Can you work these out from the model? Positions are in its coordinate system, mm. Face numbers are marked on the shaded views. A direction names the side the tool comes from. Round coordinates to 2 decimals unless told otherwise and drop trailing zeros. Loops run counter-clockwise (first coordinate to the right, second up) from the corner with the lowest first, then second, coordinate; pieces in that order, holes last. Notation, with made-up numbers: (57, 50) -> (97, 50) arc R27 ccw to (97, 83) -> close; hole circle Ø3 at (-4.5, 29.5). An arc over 180 degrees is marked (long way). Write item = value, one per line.
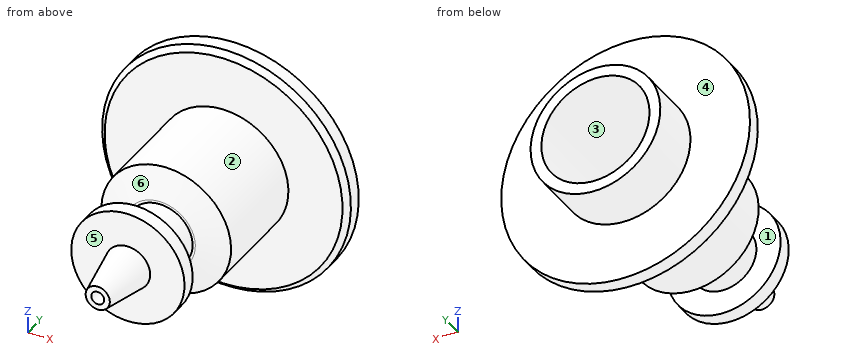
from build123d import *

# Parameters (mm, degrees)
SKETCH2_R          = 0.3
CUT_EXTRUDE1_DEPTH = 17.038105375
SKETCH2_3_R        = 2.5
SKETCH2_3_R_2      = 0.3
CUT_EXTRUDE2_DEPTH = 7.5


with BuildPart() as part:
    # Sketch1 → Revolve1 (revolve)
    with BuildSketch(Plane.XY, mode=Mode.PRIVATE) as revolve1_sk:
        Polygon((-3, 11.528571429), (-3, 9.028571429), (-5.75, 9.028571429), (-5.75, 8.378571429), (-5.5, 8.128571429), (-3, 8.128571429), (-3, 3.378571429), (-1.62626129, 2.878571429), (-1.5, 2.878571429), (-1.5, 0.878571429), (-2.618482429, 0.878571429), (-2.618482429, 0.203307318), (-1.03161177, 0.203307318), (-0.558926893, -2.29516989), (0, -2.29516989), (0, 11.528571429), align=None)
    revolve(revolve1_sk.sketch.rotate(Axis((0, 11.528571429, 0), (0, -1, 0)), 270), axis=Axis((0, 11.528571429, 0), (0, -1, 0)))

    # Sketch2 → Cut-Extrude1 (cut, through all)
    with BuildSketch(Plane(origin=(0, 11.528571429, 0), x_dir=(1, 0, 0), z_dir=(0, 1, 0))):
        with Locations(Location((0, 0, 0), (0, 0, 270))):
            Circle(SKETCH2_R)
    extrude(amount=-CUT_EXTRUDE1_DEPTH, mode=Mode.SUBTRACT)

    # Sketch2<3> → Cut-Extrude2 (cut)
    with BuildSketch(Plane(origin=(0, 11.528571429, 0), x_dir=(1, 0, 0), z_dir=(0, 1, 0))):
        with Locations(Location((0, 0, 0), (0, 0, 270))):
            Circle(SKETCH2_3_R)
        with Locations(Location((0, 0, 0), (0, 0, 270))):
            Circle(SKETCH2_3_R_2, mode=Mode.SUBTRACT)
    extrude(amount=-CUT_EXTRUDE2_DEPTH, mode=Mode.SUBTRACT)


solid = part.part
1. For the marked faces 4, 5 and 6, which set-ups out of +Z, -Z, +X, -X, +Y, -Y let a thin tool reach every point of the face, with its end or its side?
Entries:
face_4 = +Y
face_5 = -Y
face_6 = none
2. I'm going to push flat-ended pins straight in: pin 1 (4 mm diameter, centred on x = -3.5, y = 5, fed in from +Z); pin 2 (3 mm diameter, centred on x = 2, y = 4.5, fed in from +Z); pin 3 (2.5 mm diameter, centred on x = 0.5, z = 0.5, fed in from +Y). Where does each tip first touch, or does it pass through?
Entries:
pin_1 = 2.6
pin_2 = 2.96
pin_3 = 4.03
3. Suppose I cut it at A-A, the plane y = 10.5. List the corners of the cut face in (x, z) for me, and give its area (3 significant figures).
Entries:
outline = circle Ø6 at (0, 0); hole circle Ø5 at (0, 0)
area = 8.64 mm²
4. We'd pull the mould along Z, two halves only. Please class the marked faces 1, 2 and 3: released by +Z, released by -Z, zero draft, split by the parting line, or undercut.
Entries:
face_1 = zero draft
face_2 = split by the parting line
face_3 = undercut
5. I need wall thicknesses on line 1 (X direction, y = 1.5, z = 0); line 2 (X direction, y = 8.5, z = 0); line 3 (Y direction, x = -0.75, z = -4). Which ranges of each line are inside material? Lowest first, please. Write a range as [from, to].
Entries:
line_1 = [-1.5, -0.3], [0.3, 1.5]
line_2 = [-5.75, -2.5], [2.5, 5.75]
line_3 = [8.13, 9.03]
